Solid Edge part; units mm, degrees
sketch "Sketch1" plane through (0, 0, 0) normal (0, 0, 1) x (1, 0, 0)
  circle A0 centre (0, 0) radius 16
extrude "Protrusion1" add sketch "Sketch1" along normal blind 33.4
sketch "Sketch2" plane through (0, 0, 33.4) normal (0, 0, 1) x (0, 1, 0)
  circle A0 centre (0, 0) radius 16
extrude "ExtrudedProtrusion_2" add sketch "Sketch2" along normal blind 3
sketch "Sketch3" plane through (0, 0, 36.4) normal (0, 0, 1) x (1, 0, 0)
  circle A0 centre (0, 0) radius 14
extrude "ExtrudedProtrusion_3" add sketch "Sketch3" along normal blind 46.5
sketch "Sketch4" plane through (0, 0, 82.9) normal (0, 0, 1) x (0, -1, 0)
  circle A0 centre (0, 0) radius 1.5
extrude "ExtrudedProtrusion_4" add sketch "Sketch4" along normal blind 7
sketch "Sketch5" plane through (0, 0, 0) normal (0, 0, -1) x (-1, 0, 0)
  circle A0 centre (0, 0) radius 3
extrude "ExtrudedProtrusion_5" add sketch "Sketch5" along normal blind 19.3
sketch "Sketch6" plane through (0, 0, -19.3) normal (0, 0, -1) x (-1, 0, 0)
  line L0 (1.6583, 2.5) -> (-1.6583, 2.5)
  arc A0 (-1.6583, 2.5) -> (1.6583, 2.5) centre (0, 0) cw
extrude "ExtrudedCutout_1" cut sketch "Sketch6" against normal blind 12
Build history of the part. All positions in model axes, mm. A direction names the side the tool comes from. Give positions to 0.01 mm unless a question says otherwise; leave off trailing zeros. Loops run counter-clockwise (first coordinate to the right, second up) from the corner with the lowest first, then second, coordinate; pieces in that order, holes last.
Item 1: Slice it at C-C, the plane z = 27. List the corners of the cut face in (x, y), and give its area (3 significant figures).
Answers follow:
outline: circle Ø32 at (0, 0)
area: 804 mm2
Item 2: Slice it at A-A, the plane y = -8.5. List the corners of the cut face in (x, z), and give its area (3 significant figures).
Answers follow:
outline: (-13.56, 0) - (13.56, 0) - (13.56, 36.4) - (11.12, 36.4) - (11.12, 82.9) - (-11.12, 82.9) - (-11.12, 36.4) - (-13.56, 36.4) - close
area: 2,020 mm2
Item 3: Slice it at B-B, the plane x = -10.5. List the corners of the cut face in (y, z).
Answers follow:
outline: (-12.07, 0) - (12.07, 0) - (12.07, 36.4) - (9.26, 36.4) - (9.26, 82.9) - (-9.26, 82.9) - (-9.26, 36.4) - (-12.07, 36.4) - close
Item 4: Which spindle directions (+Z, -Z, +X, -X, +Y, -Y) get a long thin tool onto all of the face, cutting with end or side? Do faces 1 (the face through (0, 2.5, -13)), 2 (the face through (-0.07, 1.5, 86.35)), 3 (the face through (0, -3, -10)), 4 (the face through (0, 0, -19.3)). Say none if no direction does.
Answers follow:
face 1: -Z, +X, -X, +Y
face 2: +Z
face 3: -Z
face 4: -Z, +X, -X, +Y, -Y
Item 5: Flat gauge pins, fed straight in: pin 1 (1 mm diameter, centred on x = -5.5, y = 11.5, fed in from -Z); pin 2 (2 mm diameter, centred on x = -6, z = 34.5, fed in from -Y); pin 3 (10 mm diameter, centred on y = -3.5, z = 45, fed in from -X). Where does each tip first touch, or does it go through?
Answers follow:
pin 1: stops at z = 0
pin 2: stops at y = -15.2
pin 3: stops at x = -14
Item 6: Drill centre lines: line 1 (Z direction, x = -13, y = 4); line 2 (X direction, y = 0.5, z = 74); line 3 (Z direction, x = -11, y = 11.5). Where is each one in solid material? Low to high.
Answers follow:
line 1: z = 0 to 82.9
line 2: x = -13.99 to 13.99
line 3: z = 0 to 36.4
Item 7: Slice it at D-D, the plane z = 66.5. List the corners of the cut face in (x, y), and give its area (3 significant figures).
Answers follow:
outline: circle Ø28 at (0, 0)
area: 616 mm2
